from build123d import *

# Parameters (mm, degrees)
SKETCH1_R           = 38.1
BOSS_EXTRUDE1_DEPTH = 6.35
SKETCH2_R           = 19.05
BOSS_EXTRUDE2_DEPTH = 9.525
CUT_EXTRUDE1_START  = -9.525
CUT_EXTRUDE1_DEPTH  = 9.525
SKETCH4_R           = 6.35
CUT_EXTRUDE2_DEPTH  = 7.35
FILLET2_R           = 3.175
SKETCH7_R           = 2.38125
CUT_EXTRUDE4_DEPTH  = 6.35


with BuildPart() as part:
    # Sketch1 → Boss-Extrude1 (new body)
    with BuildSketch(Plane.XY):
        Circle(SKETCH1_R)
    extrude(amount=BOSS_EXTRUDE1_DEPTH)

    # Sketch2 → Boss-Extrude2 (add)
    with BuildSketch(Plane.XY.offset(6.35)):
        Circle(SKETCH2_R)
    extrude(amount=BOSS_EXTRUDE2_DEPTH)

    # Sketch3 → Cut-Extrude1 (cut)
    with BuildSketch(Plane(origin=(0, 0, 0), x_dir=(-1, 0, 0), z_dir=(0, 0, -1)).offset(CUT_EXTRUDE1_START)):
        with BuildLine():
            Line((-4.7625, -9.525), (4.7625, -9.525))
            ThreePointArc((4.7625, -9.525), (7.00756403, -8.59506403), (7.9375, -6.35))
            Line((7.9375, -6.35), (7.9375, 6.35))
            ThreePointArc((7.9375, 6.35), (7.00756403, 8.59506403), (4.7625, 9.525))
            Line((4.7625, 9.525), (-4.7625, 9.525))
            ThreePointArc((-4.7625, 9.525), (-7.00756403, 8.59506403), (-7.9375, 6.35))
            Line((-7.9375, 6.35), (-7.9375, -6.35))
            ThreePointArc((-7.9375, -6.35), (-7.00756403, -8.59506403), (-4.7625, -9.525))
        make_face()
    extrude(amount=CUT_EXTRUDE1_DEPTH, mode=Mode.SUBTRACT)

    # Sketch4 → Cut-Extrude2 (cut, through all)
    with BuildSketch(Plane(origin=(0, 0, 9.525), x_dir=(-1, 0, 0), z_dir=(0, 0, -1))):
        Circle(SKETCH4_R)
    extrude(amount=-CUT_EXTRUDE2_DEPTH, mode=Mode.SUBTRACT)

    # Fillet2
    fillet2_edges = [part.edges().sort_by_distance(p)[0] for p in [
        (-19.05, 0, 6.35),
    ]]
    fillet(fillet2_edges, radius=FILLET2_R)

    # Sketch7 → Cut-Extrude4 (cut)
    with BuildSketch(Plane.XY.offset(15.875)):
        with Locations((0, 12.7)):
            Circle(SKETCH7_R)
        with Locations((10.998522628, 6.35)):
            Circle(SKETCH7_R)
        with Locations((10.998522628, -6.35)):
            Circle(SKETCH7_R)
        with Locations((0, -12.7)):
            Circle(SKETCH7_R)
        with Locations((-10.998522628, -6.35)):
            Circle(SKETCH7_R)
        with Locations((-10.998522628, 6.35)):
            Circle(SKETCH7_R)
    extrude(amount=-CUT_EXTRUDE4_DEPTH, mode=Mode.SUBTRACT)


solid = part.part
Input: part model. Units: mm. Frame: model coordinates. A direction names the side the tool comes from. Give positions to 0.01 mm unless a question says otherwise; leave off trailing zeros. Order: outer loops, then holes, each group sorted by start corner. A loop starts at its lowest first (then second) coordinate and runs counter-clockwise, first axis right, second up. Notation, with made-up numbers: (30, -20) -> (46, -20) arc R19 ccw to (46, 7) -> close; hole circle Ø1 at (2.25, 65.5). An arc over 180 degrees is marked (long way). Use one line per item in the form item = value.
1) Section C-C, the plane z = 15. Return loops of the section in (x, y).
Response values:
outline = circle Ø38.1 at (0, 0); hole circle Ø4.76 at (-11, -6.35); hole circle Ø4.76 at (-11, 6.35); hole circle Ø12.7 at (0, 0); hole circle Ø4.76 at (0, -12.7); hole circle Ø4.76 at (0, 12.7); hole circle Ø4.76 at (11, -6.35); hole circle Ø4.76 at (11, 6.35)
2) Mould query, pull axis X, two halves, no side actions, for faces 4 (the cylindrical face through (-11.515, 4.025, 12.744)), 5 (the flat face through (-5, 5, 15.875)). Classes: pulls with the +X half, pulls with the -X half, needs draft (parallel to the pull), parting line crosses it, or undercut.
Response values:
face_4 = undercut
face_5 = needs draft
3) Line query: probe 1 along Y at (x, z) = (0, 13.75); probe 2 along Z at (x, y) = (-5.5, 27); probe 3 along Z at (x, y) = (0, 11) (3 decimals). Output: solid intervals per line, ascending.
Response values:
probe_1 = -19.05 to -15.08, -10.32 to -6.35, 6.35 to 10.32, 15.08 to 19.05
probe_2 = 0 to 6.35
probe_3 = 0 to 9.525
4) Section D-D, the plane y = -31. Return loops of the section in (x, z), and give its area (3 significant figures).
Response values:
outline = (-22.15, 0) -> (22.15, 0) -> (22.15, 6.35) -> (-22.15, 6.35) -> close
area = 281 mm^2
5) First-contact query: pin 1 Ø5 at (x, z) = (-0.5, 4) entering from -Y; pin 2 Ø1.5 at (y, z) = (-12.5, 1.5) entering from +X; pin 3 Ø8 at (x, z) = (-19, 12.5) entering from -Y; pin 4 Ø5 at (x, y) = (-1.5, -2) entering from -Z. Flat tips, straight axial feed; report the tip coordinate or a pass-through.
Response values:
pin_1 = -38.1
pin_2 = 36.24
pin_3 = -11.74
pin_4 = through
6) Section B-B, the plane x = 0. Return loops of the section in (y, z) (3 decimals).
Response values:
outline = (-38.1, 0) -> (-9.525, 0) -> (-9.525, 9.525) -> (-6.35, 9.525) -> (-6.35, 15.875) -> (-10.319, 15.875) -> (-10.319, 9.525) -> (-15.081, 9.525) -> (-15.081, 15.875) -> (-19.05, 15.875) -> (-19.05, 9.525) arc R3.175 cw to (-22.225, 6.35) -> (-38.1, 6.35) -> close; (6.35, 9.525) -> (9.525, 9.525) -> (9.525, 0) -> (38.1, 0) -> (38.1, 6.35) -> (22.225, 6.35) arc R3.175 cw to (19.05, 9.525) -> (19.05, 15.875) -> (15.081, 15.875) -> (15.081, 9.525) -> (10.319, 9.525) -> (10.319, 15.875) -> (6.35, 15.875) -> close
7) Reachability of faces 1 (the flat face through (-9, 1, 0)), 2 (the cylindrical face through (-9.72, -4.34, 12.74)), 3 (the flat face through (0, 9.525, 5)) from +Z, -Z, +X, -X, +Y, -Y: full face, straight path, thin tool, end or side. Return the list, or none.
Response values:
face_1 = -Z, +X, -X, +Y, -Y
face_2 = +Z
face_3 = -Z
